```python
from build123d import *

# Parameters (mm, degrees)
ESQUISSE1_W             = 140
ESQUISSE1_H             = 11
BOSS_EXTRU_1_DEPTH      = 70
ENL_V_MAT_EXTRU_1_DEPTH = 110
ESQUISSE6_W             = 30
ESQUISSE6_H             = 70
BOSS_EXTRU_3_DEPTH      = 16.4
ESQUISSE9_W             = 10
ESQUISSE9_H             = 3.5
ENL_V_MAT_EXTRU_3_DEPTH = 25
ESQUISSE10_R            = 2.25
ENL_V_MAT_EXTRU_4_DEPTH = 10.8
ESQUISSE12_W            = 110
ESQUISSE12_H            = 29
ESQUISSE12_R            = 3.05
ESQUISSE12_H_2          = 9.4
ENL_V_MAT_EXTRU_6_DEPTH = 3.8
ESQUISSE12_3_R          = 3.05
ENL_V_MAT_EXTRU_7_DEPTH = 12
BOSS_EXTRU_4_REACH      = 103.035
ESQUISSE13_W            = 110
ESQUISSE13_H            = 17.195348208


with BuildPart() as part:
    # Esquisse1 → Boss.-Extru.1 (new body)
    with BuildSketch(Plane.XY):
        Rectangle(ESQUISSE1_W, ESQUISSE1_H)
    extrude(amount=BOSS_EXTRU_1_DEPTH)

    # Esquisse2 → Enlèv. mat.-Extru.1 (cut)
    with BuildSketch(Plane.ZY.offset(70)):
        with BuildLine():
            Line((25.6, 5.5), (44.4, 5.5))
            ThreePointArc((44.4, 5.5), (35, -3.9), (25.6, 5.5))
        make_face()
    extrude(amount=-ENL_V_MAT_EXTRU_1_DEPTH, mode=Mode.SUBTRACT)

    # Esquisse6 → Boss.-Extru.3 (add)
    with BuildSketch(Plane(origin=(0, 5.5, 0), x_dir=(1, 0, 0), z_dir=(0, 1, 0))):
        with Locations((55, -35)):
            Rectangle(ESQUISSE6_W, ESQUISSE6_H)
    extrude(amount=BOSS_EXTRU_3_DEPTH)

    # Esquisse9 → Enlèv. mat.-Extru.3 (cut)
    with BuildSketch(Plane.ZY.offset(-40)):
        with Locations((35, 9.25)):
            Rectangle(ESQUISSE9_W, ESQUISSE9_H)
        with Locations((35, 20.15)):
            Rectangle(ESQUISSE9_W, ESQUISSE9_H)
    extrude(amount=-ENL_V_MAT_EXTRU_3_DEPTH, mode=Mode.SUBTRACT)

    # Esquisse10 → Enlèv. mat.-Extru.4 (cut)
    with BuildSketch(Plane(origin=(0, 18.4, 0), x_dir=(1, 0, 0), z_dir=(0, 1, 0))):
        with Locations(Location((58.15, -35, 0), (0, 0, 270))):
            Circle(ESQUISSE10_R)
        with Locations(Location((46.15, -35, 0), (0, 0, 270))):
            Circle(ESQUISSE10_R)
    extrude(amount=-ENL_V_MAT_EXTRU_4_DEPTH, mode=Mode.SUBTRACT)

    # Esquisse12 → Enlèv. mat.-Extru.6 (cut)
    # profile 1 of 3: a face of its own
    with BuildSketch(Plane(origin=(0, 5.5, 0), x_dir=(1, 0, 0), z_dir=(0, 1, 0))):
        with Locations((-15, -20.5)):
            Rectangle(ESQUISSE12_W, ESQUISSE12_H)
        with Locations(Location((30, -13, 0), (0, 0, 270))):
            Circle(ESQUISSE12_R, mode=Mode.SUBTRACT)
        with Locations(Location((-15, -13, 0), (0, 0, 270))):
            Circle(ESQUISSE12_R, mode=Mode.SUBTRACT)
        with Locations(Location((-60, -13, 0), (0, 0, 270))):
            Circle(ESQUISSE12_R, mode=Mode.SUBTRACT)
    # profile 2 of 3: a face of its own
    with BuildSketch(Plane(origin=(0, 5.5, 0), x_dir=(1, 0, 0), z_dir=(0, 1, 0))):
        with Locations((-15, -49.5)):
            Rectangle(ESQUISSE12_W, ESQUISSE12_H)
        with Locations(Location((-15, -57, 0), (0, 0, 270))):
            Circle(ESQUISSE12_R, mode=Mode.SUBTRACT)
        with Locations(Location((-60, -57, 0), (0, 0, 270))):
            Circle(ESQUISSE12_R, mode=Mode.SUBTRACT)
        with Locations(Location((30, -57, 0), (0, 0, 270))):
            Circle(ESQUISSE12_R, mode=Mode.SUBTRACT)
    # profile 3 of 3: a face of its own
    with BuildSketch(Plane(origin=(0, 5.5, 0), x_dir=(1, 0, 0), z_dir=(0, 1, 0))):
        with Locations((-15, -39.7)):
            Rectangle(ESQUISSE12_W, ESQUISSE12_H_2)
    extrude(amount=-ENL_V_MAT_EXTRU_6_DEPTH, mode=Mode.SUBTRACT)

    # Esquisse12<3> → Enlèv. mat.-Extru.7 (cut)
    with BuildSketch(Plane(origin=(0, 5.5, 0), x_dir=(1, 0, 0), z_dir=(0, 1, 0))):
        with Locations(Location((-60, -13, 0), (0, 0, 270))):
            Circle(ESQUISSE12_3_R)
        with Locations(Location((-15, -13, 0), (0, 0, 270))):
            Circle(ESQUISSE12_3_R)
        with Locations(Location((30, -13, 0), (0, 0, 270))):
            Circle(ESQUISSE12_3_R)
        with Locations(Location((30, -57, 0), (0, 0, 270))):
            Circle(ESQUISSE12_3_R)
        with Locations(Location((-60, -57, 0), (0, 0, 270))):
            Circle(ESQUISSE12_3_R)
        with Locations(Location((-15, -57, 0), (0, 0, 270))):
            Circle(ESQUISSE12_3_R)
    extrude(amount=-ENL_V_MAT_EXTRU_7_DEPTH, mode=Mode.SUBTRACT)

    # Esquisse13 → Boss.-Extru.4 (add, up to next)
    with BuildSketch(Plane(origin=(0, 1.7, 0), x_dir=(1, 0, 0), z_dir=(0, 1, 0)), mode=Mode.PRIVATE) as boss_extru_4_sk1:
        with Locations((-15, -35)):
            Rectangle(ESQUISSE13_W, ESQUISSE13_H)
    boss_extru_4_tool1 = extrude(boss_extru_4_sk1.sketch, amount=-BOSS_EXTRU_4_REACH, mode=Mode.PRIVATE) - part.part
    add(boss_extru_4_tool1.solids().sort_by_distance((-15, 1.7, 35))[0])


solid = part.part
```
Work out the finished part from the listing and answer in its coordinate system (mm). A direction names the side the tool comes from. Coordinates: 2 decimals unless noted, no trailing zeros. Loops run counter-clockwise (first coordinate to the right, second up) from the corner with the lowest first, then second, coordinate; pieces in that order, holes last. Notation, with made-up numbers: (-9.75, 75) -> (44.25, 75) arc R22 cw to (44.25, 95) -> close; hole circle Ø3 at (76, 6.5). An arc over 180 degrees is marked (long way). Answer as CSV lines item,"result".
Q1. Each of these flat-tipped pins is pushed along its axis until it touches: pin 1 (6 mm diameter, centred on y = 8.5, z = 47, fed in from -X); pin 2 (8 mm diameter, centred on x = 16, y = 11, fed in from -Z); pin 3 (4 mm diameter, centred on y = 20.5, z = 34, fed in from -X); pin 4 (10 mm diameter, centred on x = 30, z = 57, fed in from +Y). Where does it stop, or does it pass through?
Findings:
pin 1,"stops at x = 40"
pin 2,"passes through"
pin 3,"stops at x = 65"
pin 4,"stops at y = 1.7"
Q2. The part is cut by section D-D on y = 14.5. Write down the section's boundary in (x, z).
Findings:
outline,"(40, 0) -> (70, 0) -> (70, 70) -> (40, 70) -> close; hole circle Ø4.5 at (46.15, 35); hole circle Ø4.5 at (58.15, 35)"
Q3. For a pull along X with two mould halves and no side action, classify faces 1 (the face through (65, 20, 35)), 2 (the face through (52, 20, 30)), 3 (the face through (-12.94, -1.85, 10.75)) as +X half, -X half, draft (parallel to the pull), parting line (faces both ways), or undercut.
Findings:
face 1,"-X half"
face 2,"draft"
face 3,"undercut"
Q4. The part is cut by section B-B on x = -15. Write down the section's boundary in (y, z), and give its area (3 significant figures).
Findings:
outline,"(-5.5, 0) -> (5.5, 0) -> (5.5, 6) -> (1.7, 6) -> (1.7, 9.95) -> (-5.5, 9.95) -> close; (-5.5, 16.05) -> (1.7, 16.05) -> (1.7, 53.95) -> (-5.5, 53.95) -> close; (-5.5, 60.05) -> (1.7, 60.05) -> (1.7, 64) -> (5.5, 64) -> (5.5, 70) -> (-5.5, 70) -> close"
area,"462 mm²"
Q5. The part is cut by section C-C on x = 46.15. Write down the section's boundary in (y, z).
Findings:
outline,"(-5.5, 0) -> (21.9, 0) -> (21.9, 30) -> (18.4, 30) -> (18.4, 32.75) -> (11, 32.75) -> (11, 30) -> (7.5, 30) -> (7.5, 40) -> (11, 40) -> (11, 37.25) -> (18.4, 37.25) -> (18.4, 40) -> (21.9, 40) -> (21.9, 70) -> (-5.5, 70) -> close"
Q6. The part is cut by section A-A on z = 35. Write down the section's boundary in (x, y).
Findings:
outline,"(-70, -5.5) -> (70, -5.5) -> (70, 21.9) -> (65, 21.9) -> (65, 18.4) -> (60.4, 18.4) -> (60.4, 11) -> (65, 11) -> (65, 7.5) -> (40, 7.5) -> (40, 1.7) -> (-70, 1.7) -> close; (40, 11) -> (43.9, 11) -> (43.9, 18.4) -> (40, 18.4) -> close; (48.4, 11) -> (55.9, 11) -> (55.9, 18.4) -> (48.4, 18.4) -> close"
Q7. A tool of negligible diameter and unlimited length cuts with its end or side. For faces 4 (the face through (52, 20, 40)), 5 (the face through (-14.866, -1.85, 53.953)), 6 (the face through (52, 7.5, 35)), 7 (the face through (44.154, 14.752, 36.038)), from which of +Z, -Z, +X, -X, +Y, -Y can it reach the whole face along a straight path? Write none if from no direction.
Findings:
face 4,"-X, +Y"
face 5,"+Y, -Y"
face 6,"-X"
face 7,"+Y"
Q8. Find the intervals of material crossed by probe 1 along X at (y, z) = (-0.25, 57); probe 2 along X at (y, z) = (15.5, 35); probe 3 along Y at (x, z) = (51, 35), in increasing order.
Findings:
probe 1,"x = -70 to -63.05, -56.95 to -18.05, -11.95 to 26.95, 33.05 to 70"
probe 2,"x = 40 to 43.9, 48.4 to 55.9, 60.4 to 70"
probe 3,"y = -5.5 to 7.5, 11 to 18.4"
